Geometry: final body of the model. Coordinates: model frame, mm. Face numbers are marked on the shaded views. A direction names the side the tool comes from. Round coordinates to 2 decimals unless told otherwise and drop trailing zeros. Loops run counter-clockwise (first coordinate to the right, second up) from the corner with the lowest first, then second, coordinate; pieces in that order, holes last. Notation, with made-up numbers: (-16, 32.25) - (0, 32.25) arc R10 cw to (0, 47.25) - close; hole circle Ø6 at (67, 21.25). An arc over 180 degrees is marked (long way). Return JSON: item names as keys, results as strings. Group by question number.
1. Section B-B on y = -9. Return loops of the section in (x, z).
2. Material intervals for probe 1 along Y at (x, z) = (21, 6.5); probe 2 along Z at (x, y) = (7, -8); probe 3 along Z at (x, y) = (8, -1.5), sorted ascending.
3. First-contact query: pin 1 Ø4 at (y, z) = (-5, 23.5) entering from -X; pin 2 Ø7 at (x, z) = (20, 15.5) entering from +Y; pin 3 Ø1 at (y, z) = (-12, 25) entering from +X; pin 4 Ø4 at (x, y) = (12, -7) entering from +Z. Flat tips, straight axial feed; report the tip coordinate or a pass-through.
4. Section C-C on x = 10. Return loops of the section in (y, z), and give its area (3 significant figures).
5. Section D-D on y = -6.75. Return loops of the section in (x, z).
6. Section A-A on z = 15. Return loops of the section in (x, y).
7. Set-up query: the marked faces 5 and 6. Return all of +Z, -Z, +X, -X, +Y, -Y with unobstructed straight access to the full face (end or side cutting, diameter ignored); none if empty.
8. Draft query along Y for the marked faces 1, 2, 3 and 4. Return one class per face: +Y half, -Y half, draft (parallel to the pull), parting line (faces both ways), or undercut.
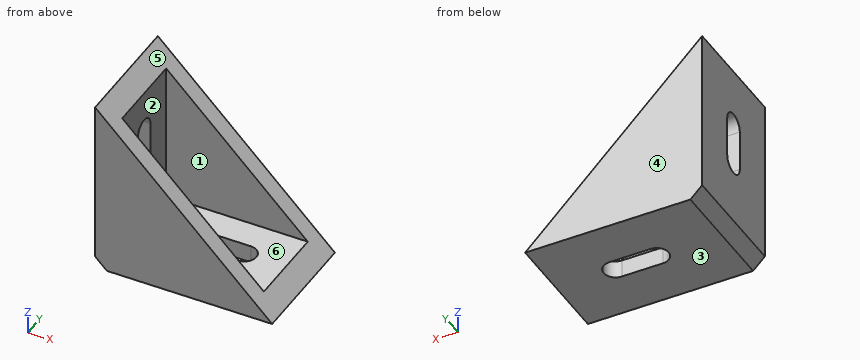
from build123d import *

# Parameters (mm, degrees)
F1_DEPTH  = 20
F3_DEPTH  = 17
F5_DEPTH  = 3
F6_SIZE   = 2
F8_DEPTH  = 25
F9_SIZE   = 2
F11_DEPTH = 25


with BuildPart() as f1:
    # F0 (on Front) → F1 (new body)
    with BuildSketch(Plane.XZ):
        Polygon((0, 30), (0, 0), (30, 0), align=None)
    extrude(amount=F1_DEPTH)

    # F2 (on Front) → F3 (cut)
    with BuildSketch(Plane.XZ):
        Polygon((29.658684, 3), (3, 28.884496), (3, 3), align=None)
    extrude(amount=F3_DEPTH, mode=Mode.SUBTRACT)

    # F4 (on face) → F5 (join)
    with BuildSketch(Plane(origin=(0, 0, 0), x_dir=(-1, 0, 0), z_dir=(0, 1, 0))):
        Polygon((-3, 3), (-3, 27), (-27, 3), align=None)
    extrude(amount=-F5_DEPTH)

    # F6
    f6_edges = [f1.edges().sort_by_distance(p)[0] for p in [
        (0, -10, 0),
    ]]
    chamfer(f6_edges, length=F6_SIZE)

    # F7 (on face) → F8 (cut)
    with BuildSketch(Plane.YZ.offset(3)):
        with BuildLine():
            ThreePointArc((-12, 20), (-10, 18), (-8, 20))
            ThreePointArc((-8, 20), (-10, 22), (-12, 20))
        make_face()
        with BuildLine():
            Line((-8, 13), (-8, 20))
            ThreePointArc((-8, 20), (-10, 18), (-12, 20))
            Line((-12, 20), (-12, 13))
            ThreePointArc((-12, 13), (-10, 15), (-8, 13))
        make_face()
        with BuildLine():
            ThreePointArc((-12, 13), (-10, 11), (-8, 13))
            ThreePointArc((-8, 13), (-10, 15), (-12, 13))
        make_face()
    extrude(amount=-F8_DEPTH, mode=Mode.SUBTRACT)

    # F9
    f9_edges = [f1.edges().sort_by_distance(p)[0] for p in [
        (3, -10, 3),
    ]]
    chamfer(f9_edges, length=F9_SIZE)

    # F10 (on face) → F11 (cut)
    with BuildSketch(Plane.XY.offset(3)):
        with BuildLine():
            ThreePointArc((20, -12), (21.414214, -11.414214), (22, -10))
            ThreePointArc((22, -10), (21.414214, -8.585786), (20, -8))
            ThreePointArc((20, -8), (18, -10), (20, -12))
        make_face()
        with BuildLine():
            ThreePointArc((20, -12), (18, -10), (20, -8))
            Line((20, -8), (13, -8))
            ThreePointArc((13, -8), (14.414214, -8.585786), (15, -10))
            ThreePointArc((15, -10), (14.414214, -11.414214), (13, -12))
            Line((13, -12), (20, -12))
        make_face()
        with BuildLine():
            ThreePointArc((15, -10), (14.414214, -8.585786), (13, -8))
            ThreePointArc((13, -8), (11, -10), (13, -12))
            ThreePointArc((13, -12), (14.414214, -11.414214), (15, -10))
        make_face()
    extrude(amount=-F11_DEPTH, mode=Mode.SUBTRACT)


solid = f1.part
Taken from the geometry:
{
 "1": {"outline": "(0, 2) - (2, 0) - (11.27, 0) - (11.27, 3) - (5, 3) - (3, 5) - (3, 11.27) - (0, 11.27) - close; (0, 21.73) - (3, 21.73) - (3, 27) - (0, 30) - close; (21.73, 0) - (30, 0) - (27, 3) - (21.73, 3) - close"},
 "2": {"probe 1": "-20 to -17, -3 to 0", "probe 2": "0 to 3", "probe 3": "0 to 22"},
 "3": {"pin 1": "x = 0", "pin 2": "through", "pin 3": "x = 3", "pin 4": "z = 3"},
 "4": {"outline": "(-20, 0) - (0, 0) - (0, 20) - (-3, 20) - (-3, 3) - (-17, 3) - (-17, 20) - (-20, 20) - close", "area": "162 mm2"},
 "5": {"outline": "(0, 2) - (2, 0) - (30, 0) - (27, 3) - (5, 3) - (3, 5) - (3, 27) - (0, 30) - close"},
 "6": {"outline": "(0, -20) - (15, -20) - (15, -17) - (3, -17) - (3, -12) - (0, -12) - close; (0, -8) - (3, -8) - (3, -3) - (15, -3) - (15, 0) - (0, 0) - close"},
 "7": {"face 5": "+Z, +X, +Y, -Y", "face 6": "+Z, +X"},
 "8": {"face 1": "undercut", "face 2": "undercut", "face 3": "draft", "face 4": "+Y half"}
}
